Verification items for the finished model (mm, model axes). A direction names the side the tool comes from. Round coordinates to 2 decimals unless told otherwise and drop trailing zeros. Order: outer loops, then holes, each group sorted by start corner. A loop starts at its lowest first (then second) coordinate and runs counter-clockwise, first axis right, second up. Notation, with made-up numbers: (61.5, 35.5) -> (85.5, 35.5) arc R11 cw to (85.5, 54.5) -> close; hole circle Ø4 at (15.25, -20.5). An arc over 180 degrees is marked (long way). Return JSON: item names as keys, results as strings. Group by question number.
1) Scan lines: L1, parallel to Z at x = -24.5, y = -5; L2, parallel to X at y = -1.5, z = 1; L3, parallel to Y at x = 23.75, z = -10.45. Record each from-to range of solid material in increasing order.
2) Draft check along X on faces 1 (the flat face through (14.26, -8.3, 4.56)), 2 (the flat face through (-12.3, 3.7, 15)), 3 (the cylindrical face through (-21, 0, -12)). Enter one of: pulls with the +X half, pulls with the -X half, needs draft (parallel to the pull), parting line crosses it, or undercut.
3) Section check D-D on x = 9. Enter the section's corners in (y, z).
4) Section check C-C on y = 7.5. Enter the section's corners in (x, z).
5) Depth check by flat-ended pin: pin 1 (10 mm diameter, centred on x = 22.5, y = -1.5, fed in from +Z); pin 2 (2 mm diameter, centred on y = -11.5, z = -1, fed in from -X); pin 3 (5 mm diameter, centred on x = -9.5, z = -10.5, fed in from -Y). Enter the tip coordinate at first touch or a pass-through.
6) Section check A-A on x = 23.75. Enter the section's corners in (y, z).
7) Tool access check on faces 4 (the cylindrical face through (0.07, 13.97, 5.9)), 5 (the cylindrical face through (-28.246, 0.198, -6.465)), 6 (the flat face through (-14.32, -8.2, 10.44)), 7 (the cylindrical face through (11.888, -7.264, 5.938)). Record the directions out of +Z, -Z, +X, -X, +Y, -Y that give a thin tool (end or side, any length) a straight path to the whole face; none if there is none.
8) Section check B-B on z = 4. Enter the section's corners in (x, y), plus the area to 3 significant figures.
```python
from build123d import *
from build123d.topology import SkipClean

# Parameters (mm, degrees)
SKETCH1_R                 = 16.5
SKETCH1_R_2               = 12.5
BOSS_EXTRUDE1_DEPTH       = 15
BOSS_EXTRUDE2_START       = 15
SKETCH2_R                 = 16.5
BOSS_EXTRUDE2_DEPTH       = 15
BOSS_EXTRUDE3_START       = -0.625485
SKETCH3_R                 = 4.5
BOSS_EXTRUDE3_DEPTH       = 0.625485
CUT_EXTRUDE1_REACH        = 41.828
CUT_EXTRUDE1_END_RADIUS   = 12.5
SKETCH4_R                 = 1.6
CIRPATTERN1_START         = -16.5
CIRPATTERN1_OUTLINE_R     = 4.5
CIRPATTERN1_OUTLINE_R_2   = 1.6
CIRPATTERN1_DEPTH         = 3.9999999
CIRPATTERN1_START_2       = 12.5000001
CIRPATTERN1_2_OUTLINE_R   = 4.5
CIRPATTERN1_2_OUTLINE_R_2 = 1.6
CIRPATTERN1_2_DEPTH       = 3.9999999
CIRPATTERN1_START_3       = -17
CIRPATTERN1_3_OUTLINE_R   = 1.6
CIRPATTERN1_3_DEPTH       = 21.886870161
CIRPATTERN1_START_4       = 12.397176997
CIRPATTERN1_4_OUTLINE_R   = 1.6
CIRPATTERN1_4_DEPTH       = 4.602823003
CHAMFER1_SIZE             = 1
SKETCH5_R                 = 2.75
BOSS_EXTRUDE4_DEPTH       = 11
SKETCH6_R                 = 4.5
CUT_EXTRUDE2_DEPTH        = 5


with BuildPart() as part:
    # Sketch1 → Boss-Extrude1 (new body)
    with BuildSketch(Plane.XY):
        Circle(SKETCH1_R)
        Circle(SKETCH1_R_2, mode=Mode.SUBTRACT)
    extrude(amount=BOSS_EXTRUDE1_DEPTH)

    # Sketch2 → Boss-Extrude2 (add)
    with BuildSketch(Plane(origin=(0, 0, 0), x_dir=(-1, 0, 0), z_dir=(0, 0, -1)).offset(BOSS_EXTRUDE2_START)):
        Circle(SKETCH2_R)
    extrude(amount=-BOSS_EXTRUDE2_DEPTH)


with BuildPart() as boss_extrude3_tool:
    # Sketch3 → Boss-Extrude3 (new body)
    with BuildSketch(Plane(origin=(0, 16.5, 0), x_dir=(1, 0, 0), z_dir=(0, 1, 0)).offset(BOSS_EXTRUDE3_START)):
        with Locations((0, -7.5)):
            Circle(SKETCH3_R)
    extrude(amount=BOSS_EXTRUDE3_DEPTH)


with BuildPart() as part_1:
    add(part.part)


with BuildPart() as part_2:
    # Boss-Extrude3: joined with boss_extrude3_tool
    add(part_1.part.fuse(boss_extrude3_tool.part, tol=0.00001))

    # Cut-Extrude1: up to this cylinder (the profile starts outside it)
    cut_extrude1_end = Plane(origin=(0, 0, 7.5), z_dir=(0, 0, -1)) * Cylinder(CUT_EXTRUDE1_END_RADIUS, 109.656, mode=Mode.PRIVATE)
    # Sketch4 → Cut-Extrude1 (cut, up to the surface)
    with BuildSketch(Plane(origin=(0, 16.5, 0), x_dir=(1, 0, 0), z_dir=(0, 1, 0)), mode=Mode.PRIVATE) as cut_extrude1_sk1:
        with Locations(Location((0, -7.5, 0), (0, 0, 270))):
            Circle(SKETCH4_R)
    cut_extrude1_tool1 = extrude(cut_extrude1_sk1.sketch, amount=-CUT_EXTRUDE1_REACH, mode=Mode.PRIVATE) - cut_extrude1_end
    add(cut_extrude1_tool1.solids().sort_by_distance((0, 16.5, 7.5))[0], mode=Mode.SUBTRACT)

    # CirPattern1: read off the stored shape, not the designer's step
    # CirPattern1 outline → CirPattern1 (add)
    with BuildSketch(Plane(origin=(0, 0, 0), x_dir=(0.500000000000004, -0.8660254037844363, 0), z_dir=(0.8660254037844363, 0.5000000000000042, 0)).offset(CIRPATTERN1_START)):
        with Locations((0, -7.5)):
            Circle(CIRPATTERN1_OUTLINE_R)
        with Locations((0, -7.5)):
            Circle(CIRPATTERN1_OUTLINE_R_2, mode=Mode.SUBTRACT)
    extrude(amount=CIRPATTERN1_DEPTH)

    # CirPattern1 2 outline → CirPattern1 2 (add)
    with BuildSketch(Plane(origin=(0, 0, 0), x_dir=(0.49999999999999195, 0.8660254037844434, 0), z_dir=(0.8660254037844433, -0.4999999999999921, 0)).offset(CIRPATTERN1_START_2)):
        with Locations((0, 7.5)):
            Circle(CIRPATTERN1_2_OUTLINE_R)
        with Locations((0, 7.5)):
            Circle(CIRPATTERN1_2_OUTLINE_R_2, mode=Mode.SUBTRACT)
    extrude(amount=CIRPATTERN1_2_DEPTH)

    # CirPattern1 3 outline → CirPattern1 3 (cut)
    with BuildSketch(Plane(origin=(0, 0, 0), x_dir=(0.500000000000004, -0.8660254037844363, 0), z_dir=(0.8660254037844363, 0.5000000000000042, 0)).offset(CIRPATTERN1_START_3)):
        with Locations((0, -7.5)):
            Circle(CIRPATTERN1_3_OUTLINE_R)
    extrude(amount=CIRPATTERN1_3_DEPTH, mode=Mode.SUBTRACT)

    # CirPattern1 4 outline → CirPattern1 4 (cut)
    with BuildSketch(Plane(origin=(0, 0, 0), x_dir=(0.49999999999999195, 0.8660254037844434, 0), z_dir=(0.8660254037844433, -0.4999999999999921, 0)).offset(CIRPATTERN1_START_4)):
        with Locations((0, 7.5)):
            Circle(CIRPATTERN1_4_OUTLINE_R)
    extrude(amount=CIRPATTERN1_4_DEPTH, mode=Mode.SUBTRACT)

    # Chamfer1
    chamfer1_edges = [part_2.edges().sort_by_distance(p)[0] for p in [
        (1.6, 16.5, 7.5),
        (-15.089419162, -6.864359354, 7.5),
        (14.855104587, -7.270204103, 8.63137085),
    ]]
    chamfer(chamfer1_edges, length=CHAMFER1_SIZE)

    # Sketch5 → Boss-Extrude4 (add)
    with SkipClean():  # the faces are left unmerged after this step: merging them gives an invalid solid
        with BuildSketch(Plane(origin=(0, 0, -15), x_dir=(-1, 0, 0), z_dir=(0, 0, -1))):
            with BuildLine():
                Line((26.573684211, 6.677522556), (6.426315789, 15.197120299))
                ThreePointArc((6.426315789, 15.197120299), (0, 16.5), (-6.426315789, 15.197120299))
                Line((-6.426315789, 15.197120299), (-26.573684211, 6.677522556))
                ThreePointArc((-26.573684211, 6.677522556), (-31, 0), (-26.573684211, -6.677522556))
                Line((-26.573684211, -6.677522556), (-6.426315789, -15.197120299))
                ThreePointArc((-6.426315789, -15.197120299), (0, -16.5), (6.426315789, -15.197120299))
                Line((6.426315789, -15.197120299), (26.573684211, -6.677522556))
                ThreePointArc((26.573684211, -6.677522556), (31, 0), (26.573684211, 6.677522556))
            make_face()
            with Locations((23.75, 0)):
                Circle(SKETCH5_R, mode=Mode.SUBTRACT)
            with Locations((-23.75, 0)):
                Circle(SKETCH5_R, mode=Mode.SUBTRACT)
        extrude(amount=-BOSS_EXTRUDE4_DEPTH)

    # Sketch6 → Cut-Extrude2 (cut)
    with SkipClean():  # the faces are left unmerged after this step: merging them gives an invalid solid
        with BuildSketch(Plane.XY.offset(-4)):
            with Locations((-23.75, 0)):
                Circle(SKETCH6_R)
            with Locations((23.75, 0)):
                Circle(SKETCH6_R)
        extrude(amount=-CUT_EXTRUDE2_DEPTH, mode=Mode.SUBTRACT)


solid = part_2.part
```
Check result:
{
 "1": {"L1": "-15 to -4", "L2": "-16.43 to -12.41, 12.41 to 16.43", "L3": "-7.87 to -2.75, 2.75 to 7.87"},
 "2": {"face 1": "pulls with the +X half", "face 2": "needs draft", "face 3": "undercut"},
 "3": {"outline": "(-14.11, -15) -> (14.11, -15) -> (14.11, -4) -> (13.83, -4) -> (13.83, 15) -> (8.67, 15) -> (8.67, 0) -> (-8.67, 0) -> (-8.67, 15) -> (-13.83, 15) -> (-13.83, -4) -> (-14.11, -4) -> close"},
 "4": {"outline": "(-24.63, -15) -> (24.63, -15) -> (24.63, -4) -> (14.7, -4) -> (14.7, 15) -> (10, 15) -> (10, 0) -> (-10, 0) -> (-10, 15) -> (-14.7, 15) -> (-14.7, -4) -> (-24.63, -4) -> close"},
 "5": {"pin 1": "z = -4", "pin 2": "x = -12.73", "pin 3": "y = -14.95"},
 "6": {"outline": "(-7.87, -15) -> (-2.75, -15) -> (-2.75, -9) -> (-4.5, -9) -> (-4.5, -4) -> (-7.87, -4) -> close; (2.75, -15) -> (7.87, -15) -> (7.87, -4) -> (4.5, -4) -> (4.5, -9) -> (2.75, -9) -> close"},
 "7": {"face 4": "+Y", "face 5": "+Z", "face 6": "+Z, -X, -Y", "face 7": "none"},
 "8": {"outline": "(-15.7, -5.8) -> (-12.88, -10.7) -> (-12.66, -10.58) arc R16.5 ccw to (12.66, -10.58) -> (12.88, -10.7) -> (15.7, -5.8) -> (15.49, -5.68) arc R16.5 ccw to (2.83, 16.26) -> (2.83, 16.5) -> (-2.83, 16.5) -> (-2.83, 16.26) arc R16.5 ccw to (-15.49, -5.68) -> close; hole circle Ø25 at (0, 0)", "area": "366 mm^2"}
}
